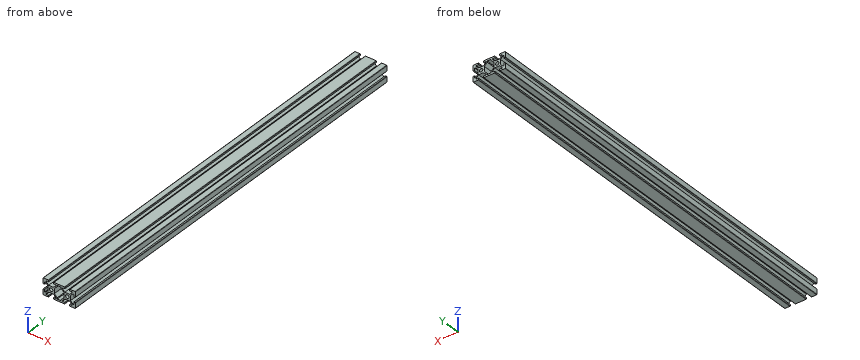
from build123d import *

# Parameters (mm, degrees)
F1_DEPTH = 500
F2_R     = 0.5


with BuildPart() as f1:
    # F0 (on Front) → F1 (new body)
    with BuildSketch(Plane.XZ):
        Polygon((-250.682858482, 19.2996120907), (-257.682858482, 19.2996120907), (-257.682858482, 12.2996120907), (-255.682858482, 12.2996120907), (-255.682858482, 15.2996120907), (-254.682858482, 15.2996120907), (-251.682858482, 12.2996120907), (-251.682858482, 13.2996120907), (-250.682858482, 13.2996120907), (-253.682858482, 16.2996120907), (-253.682858482, 17.2996120907), (-250.682858482, 17.2996120907), align=None)
        Polygon((-237.682858482, 19.2996120907), (-244.682858482, 19.2996120907), (-244.682858482, 17.2996120907), (-241.682858482, 17.2996120907), (-241.682858482, 16.2996120907), (-244.682858482, 13.2996120907), (-243.682858482, 13.2996120907), (-243.682858482, 12.2996120907), (-240.182858482, 15.7996120907), (-240.182858482, 17.2996120907), (-237.682858482, 17.2996120907), align=None)
        Polygon((-230.682858482, 19.2996120907), (-237.682858482, 19.2996120907), (-237.682858482, 17.2996120907), (-235.182858482, 17.2996120907), (-235.182858482, 15.7996120907), (-231.682858482, 12.2996120907), (-231.682858482, 13.2996120907), (-230.682858482, 13.2996120907), (-233.682858482, 16.2996120907), (-233.682858482, 17.2996120907), (-230.682858482, 17.2996120907), align=None)
        Polygon((-255.682858482, 6.2996120907), (-257.682858482, 6.2996120907), (-257.682858482, -0.7003879093), (-250.682858482, -0.7003879093), (-250.682858482, 1.2996120907), (-253.682858482, 1.2996120907), (-253.682858482, 2.2996120907), (-250.682858482, 5.2996120907), (-251.682858482, 5.2996120907), (-251.682858482, 6.2996120907), (-254.682858482, 3.2996120907), (-255.682858482, 3.2996120907), align=None)
        with BuildLine():
            ThreePointArc((-247.6828584684, 5.2996120907), (-250.5112856019, 6.4711849611), (-251.682858482, 9.2996120907))
            Line((-251.682858482, 9.2996120907), (-251.682858482, 6.2996120907))
            Line((-251.682858482, 6.2996120907), (-251.682858482, 5.2996120907))
            Line((-251.682858482, 5.2996120907), (-250.682858482, 5.2996120907))
            Line((-250.682858482, 5.2996120907), (-247.6828584684, 5.2996120907))
        make_face()
        with BuildLine():
            Line((-251.682858482, 12.2996120907), (-251.682858482, 9.2996120907))
            ThreePointArc((-251.682858482, 9.2996120907), (-250.5112856067, 12.1280392154), (-247.682858482, 13.2996120907))
            Line((-247.682858482, 13.2996120907), (-250.682858482, 13.2996120907))
            Line((-250.682858482, 13.2996120907), (-251.682858482, 13.2996120907))
            Line((-251.682858482, 13.2996120907), (-251.682858482, 12.2996120907))
        make_face()
        with BuildLine():
            Line((-249.782858482, 9.2996120907), (-251.682858482, 9.2996120907))
            ThreePointArc((-251.682858482, 9.2996120907), (-250.5112856019, 6.4711849611), (-247.6828584684, 5.2996120907))
            ThreePointArc((-247.6828584684, 5.2996120907), (-244.8544313524, 6.4711849708), (-243.682858482, 9.2996120907))
            Line((-243.682858482, 9.2996120907), (-245.582858482, 9.2996120907))
            ThreePointArc((-245.582858482, 9.2996120907), (-247.682858482, 7.1996120907), (-249.782858482, 9.2996120907))
        make_face()
        with BuildLine():
            ThreePointArc((-247.682858482, 13.2996120907), (-250.5112856067, 12.1280392154), (-251.682858482, 9.2996120907))
            Line((-251.682858482, 9.2996120907), (-249.782858482, 9.2996120907))
            ThreePointArc((-249.782858482, 9.2996120907), (-247.682858482, 11.3996120907), (-245.582858482, 9.2996120907))
            Line((-245.582858482, 9.2996120907), (-243.682858482, 9.2996120907))
            ThreePointArc((-243.682858482, 9.2996120907), (-244.8544313573, 12.1280392154), (-247.682858482, 13.2996120907))
        make_face()
        Polygon((-217.682858482, 19.2996120907), (-224.682858482, 19.2996120907), (-224.682858482, 17.2996120907), (-221.682858482, 17.2996120907), (-221.682858482, 16.2996120907), (-224.682858482, 13.2996120907), (-223.682858482, 13.2996120907), (-223.682858482, 12.2996120907), (-220.682858482, 15.2996120907), (-219.682858482, 15.2996120907), (-219.682858482, 12.2996120907), (-217.682858482, 12.2996120907), align=None)
        with BuildLine():
            Line((-244.682858482, 13.2996120907), (-247.682858482, 13.2996120907))
            ThreePointArc((-247.682858482, 13.2996120907), (-244.8544313573, 12.1280392154), (-243.682858482, 9.2996120907))
            Line((-243.682858482, 9.2996120907), (-243.682858482, 12.2996120907))
            Line((-243.682858482, 12.2996120907), (-243.682858482, 13.2996120907))
            Line((-243.682858482, 13.2996120907), (-244.682858482, 13.2996120907))
        make_face()
        with BuildLine():
            ThreePointArc((-243.682858482, 9.2996120907), (-244.8544313524, 6.4711849708), (-247.6828584684, 5.2996120907))
            Line((-247.6828584684, 5.2996120907), (-244.682858482, 5.2996120907))
            Line((-244.682858482, 5.2996120907), (-243.682858482, 5.2996120907))
            Line((-243.682858482, 5.2996120907), (-243.682858482, 6.2996120907))
            Line((-243.682858482, 6.2996120907), (-243.682858482, 9.2996120907))
        make_face()
        with BuildLine():
            ThreePointArc((-227.682858482, 5.2996120907), (-230.5112856067, 6.4711849659), (-231.682858482, 9.2996120907))
            Line((-231.682858482, 9.2996120907), (-231.682858482, 6.2996120907))
            Line((-231.682858482, 6.2996120907), (-231.682858482, 5.2996120907))
            Line((-231.682858482, 5.2996120907), (-230.682858482, 5.2996120907))
            Line((-230.682858482, 5.2996120907), (-227.682858482, 5.2996120907))
        make_face()
        with BuildLine():
            Line((-231.682858482, 12.2996120907), (-231.682858482, 9.2996120907))
            ThreePointArc((-231.682858482, 9.2996120907), (-230.5112856067, 12.1280392154), (-227.682858482, 13.2996120907))
            Line((-227.682858482, 13.2996120907), (-230.682858482, 13.2996120907))
            Line((-230.682858482, 13.2996120907), (-231.682858482, 13.2996120907))
            Line((-231.682858482, 13.2996120907), (-231.682858482, 12.2996120907))
        make_face()
        with BuildLine():
            Line((-229.782858482, 9.2996120907), (-231.682858482, 9.2996120907))
            ThreePointArc((-231.682858482, 9.2996120907), (-230.5112856067, 6.4711849659), (-227.682858482, 5.2996120907))
            ThreePointArc((-227.682858482, 5.2996120907), (-224.8544313573, 6.4711849659), (-223.682858482, 9.2996120907))
            Line((-223.682858482, 9.2996120907), (-225.582858482, 9.2996120907))
            ThreePointArc((-225.582858482, 9.2996120907), (-227.682858482, 7.1996120907), (-229.782858482, 9.2996120907))
        make_face()
        with BuildLine():
            ThreePointArc((-227.682858482, 13.2996120907), (-230.5112856067, 12.1280392154), (-231.682858482, 9.2996120907))
            Line((-231.682858482, 9.2996120907), (-229.782858482, 9.2996120907))
            ThreePointArc((-229.782858482, 9.2996120907), (-227.682858482, 11.3996120907), (-225.582858482, 9.2996120907))
            Line((-225.582858482, 9.2996120907), (-223.682858482, 9.2996120907))
            ThreePointArc((-223.682858482, 9.2996120907), (-224.8544313573, 12.1280392154), (-227.682858482, 13.2996120907))
        make_face()
        Polygon((-235.182858482, 1.2996120907), (-237.682858482, 1.2996120907), (-237.682858482, -0.7003879093), (-230.682858482, -0.7003879093), (-230.682858482, 1.2996120907), (-233.682858482, 1.2996120907), (-233.682858482, 2.2996120907), (-230.682858482, 5.2996120907), (-231.682858482, 5.2996120907), (-231.682858482, 6.2996120907), (-235.182858482, 2.7996120907), align=None)
        Polygon((-237.682858482, -0.7003879093), (-237.682858482, 1.2996120907), (-240.182858482, 1.2996120907), (-240.182858482, 2.7996120907), (-243.682858482, 6.2996120907), (-243.682858482, 5.2996120907), (-244.682858482, 5.2996120907), (-241.682858482, 2.2996120907), (-241.682858482, 1.2996120907), (-244.682858482, 1.2996120907), (-244.682858482, -0.7003879093), align=None)
        with BuildLine():
            Line((-224.682858482, 13.2996120907), (-227.682858482, 13.2996120907))
            ThreePointArc((-227.682858482, 13.2996120907), (-224.8544313573, 12.1280392154), (-223.682858482, 9.2996120907))
            Line((-223.682858482, 9.2996120907), (-223.682858482, 12.2996120907))
            Line((-223.682858482, 12.2996120907), (-223.682858482, 13.2996120907))
            Line((-223.682858482, 13.2996120907), (-224.682858482, 13.2996120907))
        make_face()
        with BuildLine():
            ThreePointArc((-223.682858482, 9.2996120907), (-224.8544313573, 6.4711849659), (-227.682858482, 5.2996120907))
            Line((-227.682858482, 5.2996120907), (-224.682858482, 5.2996120907))
            Line((-224.682858482, 5.2996120907), (-223.682858482, 5.2996120907))
            Line((-223.682858482, 5.2996120907), (-223.682858482, 6.2996120907))
            Line((-223.682858482, 6.2996120907), (-223.682858482, 9.2996120907))
        make_face()
        Polygon((-223.682858482, 5.2996120907), (-224.682858482, 5.2996120907), (-221.682858482, 2.2996120907), (-221.682858482, 1.2996120907), (-224.682858482, 1.2996120907), (-224.682858482, -0.7003879093), (-217.682858482, -0.7003879093), (-217.682858482, 6.2996120907), (-219.682858482, 6.2996120907), (-219.682858482, 3.2996120907), (-220.682858482, 3.2996120907), (-223.682858482, 6.2996120907), align=None)
    extrude(amount=F1_DEPTH)

    # F2
    f2_edges = [f1.edges().sort_by_distance(p)[0] for p in [
        (-257.682858, -250, 19.299612),
        (-250.682858, -250, 19.299612),
        (-244.682858, -250, 19.299612),
        (-230.682858, -250, 19.299612),
        (-224.682858, -250, 19.299612),
        (-217.682858, -250, 19.299612),
        (-217.682858, -250, 12.299612),
        (-217.682858, -250, 6.299612),
        (-217.682858, -250, -0.700388),
        (-230.682858, -250, -0.700388),
        (-250.682858, -250, -0.700388),
        (-257.682858, -250, 6.299612),
        (-257.682858, -250, 12.299612),
        (-257.682858, -250, -0.700388),
        (-244.682858, -250, -0.700388),
        (-224.682858, -250, -0.700388),
    ]]
    fillet(f2_edges, radius=F2_R)


solid = f1.part
Read the model definition and answer for the solid it produces. Units are mm, in the model's axes. Give positions to 0.01 mm unless a question says otherwise; leave off trailing zeros. Answer as CSV lines item,"result".
Item 1: Consider line 1 (X direction, y = -238.5, z = 1.25); line 2 (X direction, y = -166.5, z = 8.75); line 3 (Z direction, x = -227.5, y = -95.5). Determine where each line is inside the solid, lowest interval first. Write a range as [from, to].
Returned:
line 1,"x = [-257.68, -250.68], [-244.68, -230.68], [-224.68, -217.68]"
line 2,"x = [-251.68, -249.71], [-245.66, -243.68], [-231.68, -229.71], [-225.66, -223.68]"
line 3,"z = [5.3, 7.21], [11.39, 13.3]"
Item 2: Find section A-A on y = -467.5. State how many separate pieces and enclosed holes the cut face has, plus the area to 3 significant figures.
Returned:
separate pieces,"1"
enclosed holes,"3"
area,"319 mm²"
Item 3: Each of these flat-tipped pins is pushed along its axis until it touches: pin 1 (5 mm diameter, centred on x = -228, y = -250, fed in from -Z); pin 2 (2 mm diameter, centred on y = -304.5, z = 8, fed in from +X); pin 3 (2 mm diameter, centred on y = -283, z = 10.5, fed in from -X); pin 4 (3.5 mm diameter, centred on x = -227.68, z = 9.3, fed in from +Y). Where does it stop, or does it pass through?
Returned:
pin 1,"stops at z = 5.3"
pin 2,"stops at x = -223.68"
pin 3,"stops at x = -251.68"
pin 4,"passes through"
